```python
from build123d import *

# Parameters (mm, degrees)
F2_DEPTH = 40
F3_DEPTH = 8.5
F4_W     = 27
F4_H     = 30
F6_DEPTH = 110
F7_DEPTH = 30
F8_W     = 58.1251506026
F8_H     = 1.5
F9_DEPTH = 13.5


with BuildPart() as f2:
    # F0 (on Top) → F2 (new body)
    with BuildSketch(Plane.XY):
        Polygon((0, -15), (0, 0), (0, 15), (-110, 15), (-110, -15), align=None)
    extrude(amount=F2_DEPTH)

    # F0 (on Top) → F3 (cut)
    with BuildSketch(Plane.XY):
        Polygon((0, -15), (0, 0), (0, 15), (-110, 15), (-110, -15), align=None)
    extrude(amount=F3_DEPTH, mode=Mode.SUBTRACT)

    # F1 (on Front) → F5 (revolve)
    with BuildSketch(Plane.XZ):
        with BuildLine():
            Line((30.8, 0), (0, 0))
            Line((0, 0), (0, -1.5))
            Line((0, -1.5), (31, -1.5))
            ThreePointArc((31, -1.5), (43.7279220614, 3.7720779386), (49, 16.5))
            Line((49, 16.5), (49, 38.5))
            Line((49, 38.5), (54, 38.5))
            Line((54, 38.5), (54, 40))
            Line((54, 40), (47.5, 40))
            Line((47.5, 40), (47.5, 16.7))
            ThreePointArc((47.5, 16.7), (42.6086832458, 4.8913167542), (30.8, 0))
        make_face()
    revolve(axis=Axis((0, 0, -0.75), (0, 0, 1)))

    # F4 (on face) → F6 (cut)
    with BuildSketch(Plane(origin=(-110, 0, 0), x_dir=(0, -1, 0), z_dir=(-1, 0, 0))):
        with Locations((0, 25)):
            Rectangle(F4_W, F4_H)
    extrude(amount=-F6_DEPTH, mode=Mode.SUBTRACT)

    # F7 (cut): a face of the model
    f7_faces = [f2.faces().sort_by_distance(p)[0] for p in [
        (-22.4413063846, -15, 24.3086468334),
    ]]
    extrude(f7_faces, amount=-F7_DEPTH, mode=Mode.SUBTRACT)

    # F8 (on face) → F9 (cut)
    with BuildSketch(Plane.XY.offset(40)):
        with Locations((-80.9374246987, -14.25)):
            Rectangle(F8_W, F8_H)
        with Locations((-80.9374246987, 14.25)):
            Rectangle(F8_W, F8_H)
    extrude(amount=-F9_DEPTH, mode=Mode.SUBTRACT)


solid = f2.part
```
Design review of the part built by this model. Coordinates are the model's own, in mm. A direction names the side the tool comes from. Round coordinates to 2 decimals unless told otherwise and drop trailing zeros. Order: outer loops, then holes, each group sorted by start corner. A loop starts at its lowest first (then second) coordinate and runs counter-clockwise, first axis right, second up. Notation, with made-up numbers: (6, 32) - (62, 32) arc R17 cw to (62, 46) - close; hole circle Ø3 at (76, 52). An arc over 180 degrees is marked (long way). One line per question, with ' | ' between items.
Item 1: Take a section at C-C, the plane z = 2. Write out the cut boundary in (x, y), then the cut area to 3 significant figures.
Checks:
outline: circle Ø83.33 at (0, 0); hole circle Ø77.45 at (0, 0) | area: 743 mm²
Item 2: Take a section at A-A, the plane z = 18.5. Write out the cut boundary in (x, y), then the cut area to 3 significant figures.
Checks:
outline: (-110, -15) - (-46.65, -15) arc R49 ccw (long way) to (-46.65, 15) - (-110, 15) - (-110, 13.5) - (-45.07, 13.5) - (-45.07, 15) arc R47.5 cw (long way) to (-45.07, -15) - (-45.07, -13.5) - (-110, -13.5) - close | area: 604 mm²
Item 3: Wall thickness on line 1 (Y direction, x = 0, z = 32.75); line 2 (Y direction, x = -93, z = 14); line 3 (Z direction, x = -57, y = -1.5): over which ranges is each line inside the solid? List them lowest first. Write a range as [from, to].
Checks:
line 1: [-49, -47.5], [47.5, 49] | line 2: [-15, -13.5], [13.5, 15] | line 3: [8.5, 10]
Item 4: Machinability: for faces 1 (the face through (-77, -13.5, 18)), 2 (the face through (-78, -15, 17)), 3 (the face through (-77, 15, 17)), 4 (the face through (48.96, -1.94, 27.65)), which of the approach directions +Z, -Z, +X, -X, +Y, -Y give a long, thin tool a straight path to every point of the face, cutting with its end or side? Answer none if there is none.
Checks:
face 1: +Z, -X | face 2: -Z, -X, -Y | face 3: -Z, -X, +Y | face 4: -Z
Item 5: For P1, Ø1.2, axis at y = -14, z = 29.5, coming from the +X side; P2, Ø15, axis at x = -66, z = 22.5, coming from the +Y side; P3, Ø1.6, axis at x = -68, y = 14, coming from the +Z side; P4, Ø1, axis at x = -63, z = 7.5, coming from the -Y side, all flat-tipped, find the tip position at first contact; note any pin that passes through.
Checks:
P1: x = 47.13 | P2: y = 15 | P3: z = 26.5 | P4: through
Item 6: Take a section at B-B, the plane x = 0. Write out the cut boundary in (y, z), then the cut area to 3 significant figures.
Checks:
outline: (-54, 38.5) - (-49, 38.5) - (-49, 16.5) arc R18 ccw to (-31, -1.5) - (31, -1.5) arc R18 ccw to (49, 16.5) - (49, 38.5) - (54, 38.5) - (54, 40) - (47.5, 40) - (47.5, 16.7) arc R16.7 cw to (30.8, 0) - (-30.8, 0) arc R16.7 cw to (-47.5, 16.7) - (-47.5, 40) - (-54, 40) - close | area: 263 mm²
